The listing builds one solid part. Answer for the finished solid, in the listing's coordinates (mm). Coordinates: 2 decimals unless noted, no trailing zeros. Loops run counter-clockwise (first coordinate to the right, second up) from the corner with the lowest first, then second, coordinate; pieces in that order, holes last. Notation, with made-up numbers: (24, -0.75) -> (68, -0.75) arc R16 ccw to (68, 3.25) -> close; hole circle Ø4 at (66, 38.25). An arc over 180 degrees is marked (long way). Answer in a Markdown table with one row per item.
```python
from build123d import *

# Parameters (mm, degrees)
F1_DEPTH = 1800
F2_T     = -1.2


with BuildPart() as f1:
    # F0 (on Front) → F1 (new body)
    with BuildSketch(Plane.XZ):
        with BuildLine():
            ThreePointArc((0, 15), (-5.303301, 12.803301), (-7.5, 7.5))
            Line((-7.5, 7.5), (-7.5, -7.5))
            ThreePointArc((-7.5, -7.5), (-5.303301, -12.803301), (0, -15))
            ThreePointArc((0, -15), (5.303301, -12.803301), (7.5, -7.5))
            Line((7.5, -7.5), (7.5, 7.5))
            ThreePointArc((7.5, 7.5), (5.303301, 12.803301), (0, 15))
        make_face()
    extrude(amount=F1_DEPTH)

    # F2
    f2_openings = [f1.faces().sort_by_distance(p)[0] for p in [
        (0, -1800, 0),
        (0, 0, 0),
    ]]
    offset(amount=F2_T, openings=f2_openings)


solid = f1.part
```
Item 1: A cutting plane is placed at C-C, the plane x = 2.5. Determine the outline of the cut face in (y, z), plus the area to 3 significant figures.
Findings below:
| item | result |
|---|---|
| outline | (-1800, -14.57) -> (0, -14.57) -> (0, -13.28) -> (-1800, -13.28) -> close; (-1800, 13.28) -> (0, 13.28) -> (0, 14.57) -> (-1800, 14.57) -> close |
| area | 4,640 mm2 |
Item 2: A cutting plane is placed at A-A, the plane z = -1.5. Determine the outline of the cut face in (x, y).
Findings below:
| item | result |
|---|---|
| outline | (-7.5, -1800) -> (-6.3, -1800) -> (-6.3, 0) -> (-7.5, 0) -> close; (6.3, -1800) -> (7.5, -1800) -> (7.5, 0) -> (6.3, 0) -> close |
Item 3: A cutting plane is placed at B-B, the plane y = -1093.5. Determine the outline of the cut face in (x, z), plus the area to 3 significant figures.
Findings below:
| item | result |
|---|---|
| outline | (-7.5, -7.5) arc R7.5 ccw to (7.5, -7.5) -> (7.5, 7.5) arc R7.5 ccw to (-7.5, 7.5) -> close; hole (-6.3, -7.5) arc R6.3 ccw to (6.3, -7.5) -> (6.3, 7.5) arc R6.3 ccw to (-6.3, 7.5) -> close |
| area | 88.0 mm2 |
Item 4: Find the intervals of material crossed by probe 1 along X at (y, z) = (-1583, -3); probe 2 along Z at (x, y) = (0.75, -628); probe 3 along Z at (x, y) = (1.5, -527), in increasing order.
Findings below:
| item | result |
|---|---|
| probe 1 | x = -7.5 to -6.3, 6.3 to 7.5 |
| probe 2 | z = -14.96 to -13.76, 13.76 to 14.96 |
| probe 3 | z = -14.85 to -13.62, 13.62 to 14.85 |
Item 5: A flat-ended cylindrical pin translates along its axis: pin 1 Ø6 at (x, y) = (2.5, -1045.5) entering from +Z. Find the tip coordinate at first contact, or state that the pin passes through.
Findings below:
| item | result |
|---|---|
| pin 1 | stops at z = 15 |
